```python
from build123d import *
from OCP.BRepFilletAPI import BRepFilletAPI_MakeChamfer

# Parameters (mm, degrees)
SKETCH1_W           = 150
SKETCH1_H           = 100
BOSS_EXTRUDE1_DEPTH = 250
FILLET1_R           = 50
SKETCH4_W           = 15
SKETCH4_H           = 60
CUT_EXTRUDE2_DEPTH  = 6
SKETCH5_W           = 15
SKETCH5_H           = 8
CUT_EXTRUDE3_DEPTH  = 4
CHAMFER2_SIZE       = 2
CHAMFER2_SIZE2      = 3.464101615
SHELL1_START        = 42
SHELL1_OUTLINE_W    = 248
SHELL1_OUTLINE_H    = 96
SHELL1_DEPTH        = 66
SHELL1_START_2      = 2
SHELL1_2_DEPTH      = 40
SHELL1_START_3      = 108
SHELL1_3_DEPTH      = 40
SHELL1_4_DEPTH      = 21
SHELL1_START_4      = 127
SHELL1_5_DEPTH      = 21
SHELL1_6_DEPTH      = 250
FILLET4_R           = 6
SKETCH6_W           = 10
SKETCH6_H           = 3
EXTRUDE_THIN1_DEPTH = 9.5
FILLET5_R           = 3
CUT_EXTRUDE4_REACH  = 304.212
SKETCH7_R           = 3
FILLET6_R           = 0.5
SKETCH8_R           = 3
CUT_EXTRUDE5_DEPTH  = 10


with BuildPart() as part:
    # Sketch1 → Boss-Extrude1 (new body)
    with BuildSketch(Plane(origin=(0, 0, 0), x_dir=(1, 0, 0), z_dir=(0, 1, 0))):
        with Locations((75, 50)):
            Rectangle(SKETCH1_W, SKETCH1_H)
    extrude(amount=BOSS_EXTRUDE1_DEPTH)

    # Fillet1
    fillet1_edges = [part.edges().sort_by_distance(p)[0] for p in [
        (0, 125, -100),
        (150, 125, -100),
    ]]
    fillet(fillet1_edges, radius=FILLET1_R)

    # Sketch4 → Cut-Extrude2 (cut)
    with BuildSketch(Plane.XZ):
        with Locations((32.5, -30)):
            Rectangle(SKETCH4_W, SKETCH4_H)
        with Locations((117.5, -30)):
            Rectangle(SKETCH4_W, SKETCH4_H)
    extrude(amount=-CUT_EXTRUDE2_DEPTH, mode=Mode.SUBTRACT)

    # Sketch5 → Cut-Extrude3 (cut)
    with BuildSketch(Plane.XZ.offset(-6)):
        with Locations((32.5, -12)):
            Rectangle(SKETCH5_W, SKETCH5_H)
        with Locations((117.5, -12)):
            Rectangle(SKETCH5_W, SKETCH5_H)
    extrude(amount=-CUT_EXTRUDE3_DEPTH, mode=Mode.SUBTRACT)

    # Chamfer2: one chamfer whose edges measure the first distance from different faces: ONE call of the kernel's chamfer builder (chamfer() names one face for all edges)
    chamfer2_edges_1 = [part.edges().sort_by_distance(p)[0] for p in [
        (32.5, 6, -16),
    ]]
    chamfer2_side_1 = [part.faces().sort_by_distance(p)[0] for p in [
        (32.5, 6, -38),
    ]]
    chamfer2_edges_2 = [part.edges().sort_by_distance(p)[0] for p in [
        (32.5, 6, -8),
    ]]
    chamfer2_side_2 = [part.faces().sort_by_distance(p)[0] for p in [
        (32.5, 6, -4),
    ]]
    chamfer2_edges_3 = [part.edges().sort_by_distance(p)[0] for p in [
        (117.5, 6, -16),
    ]]
    chamfer2_side_3 = [part.faces().sort_by_distance(p)[0] for p in [
        (117.5, 6, -38),
    ]]
    chamfer2_edges_4 = [part.edges().sort_by_distance(p)[0] for p in [
        (117.5, 6, -8),
    ]]
    chamfer2_side_4 = [part.faces().sort_by_distance(p)[0] for p in [
        (117.5, 6, -4),
    ]]
    chamfer2 = BRepFilletAPI_MakeChamfer(part.part.solid().wrapped)
    for e in chamfer2_edges_1:
        chamfer2.Add(CHAMFER2_SIZE, CHAMFER2_SIZE2, e.wrapped, chamfer2_side_1[0].wrapped)  # the first distance lies on this face
    for e in chamfer2_edges_2:
        chamfer2.Add(CHAMFER2_SIZE, CHAMFER2_SIZE2, e.wrapped, chamfer2_side_2[0].wrapped)  # the first distance lies on this face
    for e in chamfer2_edges_3:
        chamfer2.Add(CHAMFER2_SIZE, CHAMFER2_SIZE2, e.wrapped, chamfer2_side_3[0].wrapped)  # the first distance lies on this face
    for e in chamfer2_edges_4:
        chamfer2.Add(CHAMFER2_SIZE, CHAMFER2_SIZE2, e.wrapped, chamfer2_side_4[0].wrapped)  # the first distance lies on this face
    add(Compound.cast(chamfer2.Shape()), mode=Mode.REPLACE)

    # Shell1: read off the stored shape, not the designer's step
    # Shell1 outline → Shell1 (cut)
    with BuildSketch(Plane.YZ.offset(SHELL1_START)):
        with Locations((126, -50)):
            Rectangle(SHELL1_OUTLINE_W, SHELL1_OUTLINE_H)
    extrude(amount=SHELL1_DEPTH, mode=Mode.SUBTRACT)

    # Shell1 2 outline → Shell1 2 (cut)
    with BuildSketch(Plane.YZ.offset(SHELL1_START_2)):
        Polygon((8, -2), (8, -4.845299462), (10, -6), (12, -6), (12, -18), (10, -18), (8, -19.154700538), (8, -62), (2, -62), (2, -98), (250, -98), (250, -2), align=None)
    extrude(amount=SHELL1_2_DEPTH, mode=Mode.SUBTRACT)

    # Shell1 3 outline → Shell1 3 (cut)
    with BuildSketch(Plane.YZ.offset(SHELL1_START_3)):
        Polygon((8, -2), (8, -4.845299462), (10, -6), (12, -6), (12, -18), (10, -18), (8, -19.154700538), (8, -62), (2, -62), (2, -98), (250, -98), (250, -2), align=None)
    extrude(amount=SHELL1_3_DEPTH, mode=Mode.SUBTRACT)

    # Shell1 4 outline → Shell1 4 (cut)
    with BuildSketch(Plane.YZ.offset(SHELL1_START_2)):
        Polygon((10, -6), (8, -4.845299462), (8, -2), (2, -2), (2, -62), (8, -62), (8, -19.154700538), (10, -18), (12, -18), (12, -6), align=None)
    extrude(amount=SHELL1_4_DEPTH, mode=Mode.SUBTRACT)

    # Shell1 5 outline → Shell1 5 (cut)
    with BuildSketch(Plane.YZ.offset(SHELL1_START_4)):
        Polygon((10, -6), (8, -4.845299462), (8, -2), (2, -2), (2, -62), (8, -62), (8, -19.154700538), (10, -18), (12, -18), (12, -6), align=None)
    extrude(amount=SHELL1_5_DEPTH, mode=Mode.SUBTRACT)

    # Shell1 6 outline → Shell1 6 (add)
    with BuildSketch(Plane(origin=(0, 0, 0), x_dir=(1, 0, 0), z_dir=(0, 1, 0))):
        with BuildLine():
            Line((114, 98), (100, 98))
            ThreePointArc((100, 98), (133.941125497, 83.941125497), (148, 50))
            Line((148, 50), (148, 64))
            ThreePointArc((148, 64), (135.355339059, 85.355339059), (114, 98))
        make_face()
        with BuildLine():
            ThreePointArc((36, 98), (14.644660941, 85.355339059), (2, 64))
            Line((2, 64), (2, 50))
            ThreePointArc((2, 50), (16.058874503, 83.941125497), (50, 98))
            Line((50, 98), (36, 98))
        make_face()
    extrude(amount=SHELL1_6_DEPTH)

    # Fillet4
    fillet4_edges = [part.edges().sort_by_distance(p)[0] for p in [
        (12.5, 2, -2),
        (2, 2, -26),
        (16.058874503, 2, -83.941125497),
        (75, 2, -98),
        (133.941125497, 2, -83.941125497),
        (148, 2, -26),
        (137.5, 2, -2),
        (108, 2, -32),
        (127, 2, -32),
        (117.5, 2, -62),
        (75, 2, -2),
        (23, 2, -32),
        (42, 2, -32),
        (32.5, 2, -62),
        (2, 126, -2),
        (148, 126, -2),
    ]]
    fillet(fillet4_edges, radius=FILLET4_R - 0.0001)  # a hair under: the kernel refuses the full size

    # Sketch6 → Extrude-Thin1 (add)
    with BuildSketch(Plane(origin=(0, 2, 0), x_dir=(1, 0, 0), z_dir=(0, 1, 0))):
        with Locations((72, 81.075172512)):
            Rectangle(SKETCH6_W, SKETCH6_H)
    extrude(amount=EXTRUDE_THIN1_DEPTH)

    # Fillet5
    fillet5_edges = [part.edges().sort_by_distance(p)[0] for p in [
        (72, 2, -79.575172512),
        (67, 2, -81.075172512),
        (72, 2, -82.575172512),
        (77, 2, -81.075172512),
    ]]
    fillet(fillet5_edges, radius=FILLET5_R)

    # Sketch7 → Cut-Extrude4 (cut, up to next)
    with BuildSketch(Plane.XY.offset(-79.575172512), mode=Mode.PRIVATE) as cut_extrude4_sk1:
        with Locations((72, 9)):
            Circle(SKETCH7_R)
    cut_extrude4_tool1 = extrude(cut_extrude4_sk1.sketch, amount=-CUT_EXTRUDE4_REACH, mode=Mode.PRIVATE) & part.part
    add(cut_extrude4_tool1.solids().sort_by_distance((72, 9, -79.575173))[0], mode=Mode.SUBTRACT)

    # Fillet6
    fillet6_edges = [part.edges().sort_by_distance(p)[0] for p in [
        (73.658312395, 11.5, -81.075172512),
        (70.341687605, 11.5, -81.075172512),
    ]]
    fillet(fillet6_edges, radius=FILLET6_R)

    # Sketch8 → Cut-Extrude5 (cut)
    with BuildSketch(Plane(origin=(0, 0, -2), x_dir=(-1, 0, 0), z_dir=(0, 0, -1))):
        with Locations((-25, 241)):
            Circle(SKETCH8_R)
    extrude(amount=-CUT_EXTRUDE5_DEPTH, mode=Mode.SUBTRACT)


solid = part.part
```
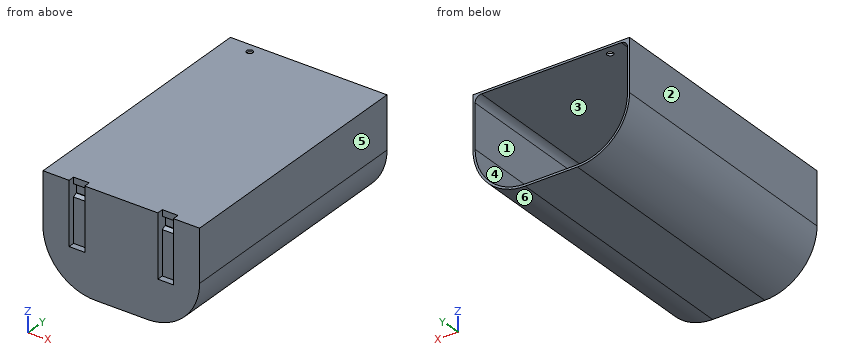
Check sheet for the modelled part. Datum: model origin and axes. Units: mm. Face numbers are marked on the shaded views. A direction names the side the tool comes from. Give positions to 0.01 mm unless a question says otherwise; leave off trailing zeros. Write each loop counter-clockwise with the first axis right and the second up, starting at its lowest first coordinate (ties: lowest second). Pieces come first, ordered by that corner, then holes.
Item 1: Cross-section at A-A (y = 241). Enter the section's corners in (x, z).
Item 2: Cross-section at B-B (y = 199). Enter the section's corners in (x, z).
Item 3: Scan lines: L1, parallel to X at y = 75.5, z = -19; L2, parallel to Z at x = 89, y = 44.5; L3, parallel to X at y = 241, z = -1. Record each from-to range of solid material in increasing order.
Item 4: Draft check along Z on the marked faces 3, 4, 5 and 6. Enter one of: released by +Z, released by -Z, zero draft, split by the parting line, or undercut.
Item 5: Gauge pin test, flat ends, axial feed: pin 1 (5 mm diameter, centred on x = 106.5, z = -68.5, fed in from -Y); pin 2 (1 mm diameter, centred on x = 126, z = -63.5, fed in from +Y); pin 3 (8 mm diameter, centred on x = 17, y = 78, fed in from -Z); pin 4 (5 mm diameter, centred on x = 34.5, y = 1.5, fed in from +Z). Record the tip position at first contact, or that the pin passes through.
Item 6: Access from +Z, -Z, +X, -X, +Y, -Y to the whole of each face (thin tool, end or side, straight path). Record for the marked faces 1 and 2.
Report:
1. outline: (0, -50) arc R50 ccw to (50, -100) - (100, -100) arc R50 ccw to (150, -50) - (150, 0) - (28, 0) - (28, -2) - (142, -2) arc R6 cw to (148, -8) - (148, -50) arc R48 cw to (100, -98) - (50, -98) arc R48 cw to (2, -50) - (2, -8) arc R6 cw to (8, -2) - (22, -2) - (22, 0) - (0, 0) - close
2. outline: (0, -50) arc R50 ccw to (50, -100) - (100, -100) arc R50 ccw to (150, -50) - (150, 0) - (0, 0) - close; hole (2, -50) arc R48 ccw to (50, -98) - (100, -98) arc R48 ccw to (148, -50) - (148, -8) arc R6 ccw to (142, -2) - (8, -2) arc R6 ccw to (2, -8) - close
3. L1: x = 0 to 2, 148 to 150
3. L2: z = -100 to -98, -2 to 0
3. L3: x = 0 to 22, 28 to 150
4. face 3: undercut
4. face 4: undercut
4. face 5: zero draft
4. face 6: released by -Z
5. pin 1: stops at y = 0
5. pin 2: stops at y = 4.68
5. pin 3: stops at z = -90.73
5. pin 4: stops at z = -60
6. face 1: +Y
6. face 2: +Z, -Z, -X, +Y, -Y
